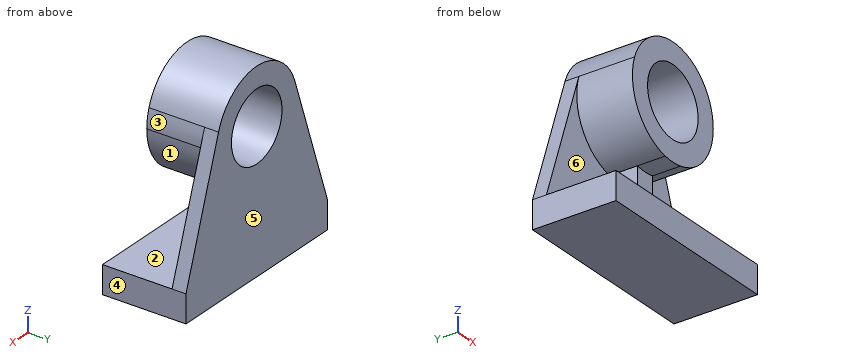
```python
from build123d import *

# Parameters (mm, degrees)
F0_R     = 63.5
F1_DEPTH = 127
F2_DEPTH = 152.4
F3_DEPTH = 76.2
F4_DEPTH = 25.4


with BuildPart() as f1:
    # F0 (on Front) → F1 (new body)
    with BuildSketch(Plane.XZ):
        with BuildLine():
            ThreePointArc((19.05, -99.798084), (78.288058, -64.757548), (101.6, 0))
            ThreePointArc((101.6, 0), (100.194597, 16.840506), (96.017271, 33.215112))
            ThreePointArc((96.017271, 33.215112), (0, 101.6), (-96.017271, 33.215112))
            ThreePointArc((-96.017271, 33.215112), (-87.938881, -50.885295), (-19.05, -99.798084))
            ThreePointArc((-19.05, -99.798084), (0, -101.6), (19.05, -99.798084))
        make_face()
        Circle(F0_R, mode=Mode.SUBTRACT)
    extrude(amount=F1_DEPTH)



with BuildPart() as f2:
    # F0 (on Front) → F2 (new body)
    with BuildSketch(Plane.XZ):
        Polygon((177.8, -254), (177.8, -203.2), (19.05, -203.2), (-19.05, -203.2), (-177.8, -203.2), (-177.8, -254), align=None)
    extrude(amount=F2_DEPTH)


with BuildPart() as f1_1:
    add(f1.part)

    add(f2.part)  # F3 merges F2
    # F0 (on Front) → F3 (join)
    with BuildSketch(Plane.XZ):
        with BuildLine():
            Line((19.05, -203.2), (19.05, -99.798084))
            ThreePointArc((19.05, -99.798084), (0, -101.6), (-19.05, -99.798084))
            Line((-19.05, -99.798084), (-19.05, -203.2))
            Line((-19.05, -203.2), (19.05, -203.2))
        make_face()
    extrude(amount=F3_DEPTH)

    # F0 (on Front) → F4 (join)
    with BuildSketch(Plane.XZ):
        with BuildLine():
            ThreePointArc((-19.05, -99.798084), (-87.938881, -50.885295), (-96.017271, 33.215112))
            Line((-96.017271, 33.215112), (-177.8, -203.2))
            Line((-177.8, -203.2), (-19.05, -203.2))
            Line((-19.05, -203.2), (-19.05, -99.798084))
        make_face()
        with BuildLine():
            ThreePointArc((96.017271, 33.215112), (100.194597, 16.840506), (101.6, 0))
            ThreePointArc((101.6, 0), (78.288058, -64.757548), (19.05, -99.798084))
            Line((19.05, -99.798084), (19.05, -203.2))
            Line((19.05, -203.2), (177.8, -203.2))
            Line((177.8, -203.2), (96.017271, 33.215112))
        make_face()
    extrude(amount=F4_DEPTH)


solid = f1_1.part
```
For this review, take the finished solid that the model builds, in its own axes (mm). Face numbers are marked on the shaded views. A direction names the side the tool comes from. Round coordinates to 2 decimals unless told otherwise and drop trailing zeros. Write each loop counter-clockwise with the first axis right and the second up, starting at its lowest first coordinate (ties: lowest second). Pieces come first, ordered by that corner, then holes. Notation, with made-up numbers: (48, -14) - (103, -14) arc R13 cw to (103, 1) - close; hole circle Ø2 at (-2.75, 30.25). An arc over 180 degrees is marked (long way). Use CSV: the item, a comma, the result in double quotes.
1) Add section A-A on x = 0. Write out the cut boundary in (y, z).
Conclusion:
outline,"(-152.4, -254) - (0, -254) - (0, -63.5) - (-127, -63.5) - (-127, -101.6) - (-76.2, -101.6) - (-76.2, -203.2) - (-152.4, -203.2) - close; (-127, 63.5) - (0, 63.5) - (0, 101.6) - (-127, 101.6) - close"
2) Wall thickness on line 1 along Z through (x, y) = (0, -91.5); line 2 along Z through (x, y) = (0, -66); line 3 along Z through (x, y) = (52.5, -102.5): over which ranges is each line inside the solid? List them lowest first. Write a range as from..to.
Conclusion:
line 1,"z = -254..-203.2, -101.6..-63.5, 63.5..101.6"
line 2,"z = -254..-63.5, 63.5..101.6"
line 3,"z = -254..-203.2, -86.98..-35.72, 35.72..86.98"
3) The part is to be moulded in two halves that separate along Y. For the marked faces 4, 5 and 6, say which applies: pulls with the +Y half, pulls with the -Y half, needs draft (parallel to the pull), parting line crosses it, or undercut.
Conclusion:
face 4,"needs draft"
face 5,"pulls with the +Y half"
face 6,"pulls with the -Y half"
4) Add section C-C on x = -69.5. Write out the cut boundary in (y, z), and give its area (3 significant figures).
Conclusion:
outline,"(-152.4, -254) - (0, -254) - (0, 74.11) - (-127, 74.11) - (-127, -74.11) - (-25.4, -74.11) - (-25.4, -203.2) - (-152.4, -203.2) - close"
area,"29,800 mm^2"
5) Add section B-B on y = -9.5. Write out the cut boundary in (x, z), and give its area (3 significant figures).
Conclusion:
outline,"(-177.8, -254) - (177.8, -254) - (177.8, -203.2) - (96.02, 33.22) arc R101.6 ccw to (-96.02, 33.22) - (-177.8, -203.2) - close; hole circle Ø127 at (0, 0)"
area,"79,700 mm^2"
6) For the marked faces 1, 2 and 3, list the 3-axis set-ups (+Z, -Z, +X, -X, +Y, -Y) from which the entire face can be reached by the end or side of a thin tool; tool diameter is ignored.
Conclusion:
face 1,"+X, -Y"
face 2,"-Y"
face 3,"+Z, +X, -Y"
7) Clearance check with flat-ended pins moving along their axes: pin 1 Ø5 at (y, z) = (-15.5, -47) entering from +X; pin 2 Ø1 at (y, z) = (-18, -197) entering from -X; pin 3 Ø15 at (y, z) = (-45.5, -130.5) entering from +X. State where each tip first meets the part, or that it passes through.
Conclusion:
pin 1,"stops at x = 124.63"
pin 2,"stops at x = -175.83"
pin 3,"stops at x = 19.05"
8) Add section D-D on z = -156. Write out the cut boundary in (x, y).
Conclusion:
outline,"(-161.47, -25.4) - (-19.05, -25.4) - (-19.05, -76.2) - (19.05, -76.2) - (19.05, -25.4) - (161.47, -25.4) - (161.47, 0) - (-161.47, 0) - close"
